```python
from build123d import *

# Parameters (mm, degrees)
SKETCH1_W           = 152.4
SKETCH1_H           = 37
BOSS_EXTRUDE1_DEPTH = 101.6
SKETCH2_W           = 99.6
SKETCH2_H           = 35
CUT_EXTRUDE1_DEPTH  = 185.093916249
SKETCH3_W           = 150.4
SKETCH3_H           = 99.6
CUT_EXTRUDE2_DEPTH  = 133.280006048
EXTRUDE_THIN4_START = -101.6
EXTRUDE_THIN4_DEPTH = 101.6
SKETCH9_W           = 106.403135183
SKETCH9_H           = 5
BOSS_EXTRUDE4_DEPTH = 101.6


# Read off the part's stored shape, not the designer's step: Extrude-Thin4
with BuildPart() as part:
    # Sketch1 → Boss-Extrude1 (new body)
    with BuildSketch(Plane.XY):
        Rectangle(SKETCH1_W, SKETCH1_H)
    extrude(amount=BOSS_EXTRUDE1_DEPTH)

    # Sketch2 → Cut-Extrude1 (cut, through all)
    with BuildSketch(Plane.ZY.offset(76.2)):
        with Locations((50.8, 0)):
            Rectangle(SKETCH2_W, SKETCH2_H)
    extrude(amount=-CUT_EXTRUDE1_DEPTH, mode=Mode.SUBTRACT)

    # Sketch3 → Cut-Extrude2 (cut, through all)
    with BuildSketch(Plane(origin=(0, 18.5, 0), x_dir=(1, 0, 0), z_dir=(0, 1, 0))):
        with Locations((0, -50.8)):
            Rectangle(SKETCH3_W, SKETCH3_H)
    extrude(amount=-CUT_EXTRUDE2_DEPTH, mode=Mode.SUBTRACT)

    # Extrude-Thin4 outline → Extrude-Thin4 (add)
    with BuildSketch(Plane(origin=(0, 0, 0), x_dir=(-1, 0, 0), z_dir=(0, 0, -1)).offset(EXTRUDE_THIN4_START)):
        with BuildLine():
            Line((-76.2, 43.5), (-76.2, 18.5))
            Line((-76.2, 18.5), (40.203135183, 18.5))
            Line((40.203135183, 18.5), (40.203135183, 28.5))
            Line((40.203135183, 28.5), (-66.2, 28.5))
            Line((-66.2, 28.5), (-66.2, 33.5))
            Line((-66.2, 33.5), (37.076687279, 33.5))
            add(Edge.make_bspline(
                [(37.076687279, 33.5), (42.712503235, 29.602755941), (47.740101517, 26.184011055), (56.600294641, 20.291071098), (60.430190038, 17.818058565), (65.330997145, 14.789830611), (66.824161054, 13.89378122), (69.560877297, 12.31480535), (70.801570346, 11.632483882), (72.54251455, 10.745567395), (73.103276521, 10.472479574), (74.21882377, 9.963704392), (74.771996239, 9.727837773), (75.629792754, 9.404385606), (75.906990567, 9.305691485), (76.2, 9.210010654)],
                knots=[0, 0, 0, 0, 0.25, 0.25, 0.5, 0.5, 0.625, 0.625, 0.75, 0.75, 0.8125, 0.8125, 0.875, 0.875, 0.903624295, 0.903624295, 0.903624295, 0.903624295], degree=3))
            add(Edge.make_bspline(
                [(76.2, 9.210010654), (76.22687774, 9.201233856), (76.253888525, 9.192482414), (76.604166758, 9.079903255), (76.946677128, 8.979439764), (77.707610171, 8.79063089), (78.125422966, 8.701549246), (79.103306411, 8.557457163), (79.663066468, 8.499997568), (80.351085446, 8.499997395)],
                knots=[0.903624295, 0.903624295, 0.903624295, 0.903624295, 0.90625, 0.90625, 0.9375, 0.9375, 0.96875, 0.96875, 1, 1, 1, 1], degree=3))
            Line((80.351085446, 8.499997395), (80.351087966, 18.499997395))
            add(Edge.make_bspline(
                [(40.203135183, 43.5), (76.200002245, 18.499998441), (80.351087966, 18.499997395)],
                knots=[0, 0, 0, 1, 1, 1], degree=2))
            Line((40.203135183, 43.5), (-76.2, 43.5))
        make_face()
    extrude(amount=EXTRUDE_THIN4_DEPTH)

    # Sketch9 → Boss-Extrude4 (add)
    with BuildSketch(Plane(origin=(0, 0, 0), x_dir=(-1, 0, 0), z_dir=(0, 0, -1))):
        with Locations((-12.998432409, 31)):
            Rectangle(SKETCH9_W, SKETCH9_H)
    extrude(amount=-BOSS_EXTRUDE4_DEPTH)


solid = part.part
```
For this review, take the finished solid that the model builds, in its own axes (mm). Coordinates: 2 decimals unless noted, no trailing zeros. Order: outer loops, then holes, each group sorted by start corner. A loop starts at its lowest first (then second) coordinate and runs counter-clockwise, first axis right, second up. Notation, with made-up numbers: (65.25, 53.25) -> (69.25, 53.25) arc R5 cw to (69.25, 58.25) -> close; hole circle Ø6 at (27, 17.25). An arc over 180 degrees is marked (long way). Use CSV: the item, a comma, the result in double quotes. Start each with the question number.
Item 1: We need section A-A, the plane y = 0. Give the boundary of the cut face in (x, z), then the cut area to 3 significant figures.
Item 2: We need section C-C, the plane z = 90. Give the number of separate pieces and of enclosed holes in the cut face, then the cut area to 3 significant figures.
Item 3: Wall thickness on probe 1 along Z at (x, y) = (28, 4); probe 2 along Y at (x, z) = (31, 76); probe 3 along X at (y, z) = (30, 21.5): over which ranges is each line inside the solid? List them lowest first.
Item 4: Insertion check: pin 1 (6 mm diameter, centred on y = 30, z = 54, fed in from -X); pin 2 (22 mm diameter, centred on y = -8, z = 29.5, fed in from -X); pin 3 (0.5 mm diameter, centred on x = -45, z = 0.5, fed in from +Y). Each pin has a flat end and moves straight along its axis. Give the tip position at first contact, or say it passes through.
Item 5: Draft analysis for pull direction X (two halves, no side actions). For faces 1 (the face through (76.2, 34, 52)), 2 (the face through (-1, 13, 0)), 3 (the face through (-80.351, 13, 52)), 4 (the face through (18, 18.5, 51)), state which applies: pulls with the +X half, pulls with the -X half, needs draft (parallel to the pull), parting line crosses it, or undercut.
Item 6: We need section B-B, the plane x = 0. Give the boundary of the cut face in (y, z).
Derived:
1,outline,"(-76.2, 0) -> (76.2, 0) -> (76.2, 1) -> (-76.2, 1) -> close; (-76.2, 100.6) -> (76.2, 100.6) -> (76.2, 101.6) -> (-76.2, 101.6) -> close"
1,area,"305 mm^2"
2,separate pieces,"3"
2,enclosed holes,"0"
2,area,"3,380 mm^2"
3,probe 1,"z = 0 to 1, 100.6 to 101.6"
3,probe 2,"y = 18.5 to 43.5"
3,probe 3,"x = -60.07 to -42.16, -40.2 to 76.2"
4,pin 1,"stops at x = -64.68"
4,pin 2,"stops at x = -76.2"
4,pin 3,"stops at y = 40.35"
5,face 1,"pulls with the +X half"
5,face 2,"needs draft"
5,face 3,"pulls with the -X half"
5,face 4,"undercut"
6,outline,"(-18.5, 0) -> (43.5, 0) -> (43.5, 101.6) -> (-18.5, 101.6) -> (-18.5, 100.6) -> (18.5, 100.6) -> (18.5, 1) -> (-18.5, 1) -> close"
